```python
from build123d import *

# Parameters (mm, degrees)
SKETCH1_R           = 2.75
BOSS_EXTRUDE1_DEPTH = 6.35


with BuildPart() as part:
    # Sketch1 → Boss-Extrude1 (new body)
    with BuildSketch(Plane.XY):
        Polygon((182, -212), (212, -212), (212, -182), (232.5, -182), (232.5, 0), (232.5, 182), (212, 182), (212, 212), (182, 212), (182, 232.5), (8, 232.5), (8, 191.5), (-48, 191.5), (-48, 232.5), (-182, 232.5), (-182, 212), (-212, 212), (-212, 182), (-232.5, 182), (-232.5, 0), (-232.5, -182), (-212, -182), (-212, -212), (-182, -212), (-182, -232.5), (-8, -232.5), (-8, -191.5), (48, -191.5), (48, -232.5), (182, -232.5), align=None)
        with Locations((-222.5, -162)):
            Circle(SKETCH1_R, mode=Mode.SUBTRACT)
        with Locations(Location((222.5, -162, 0), (0, 0, 180))):
            Circle(SKETCH1_R, mode=Mode.SUBTRACT)
        with Locations((222.5, 162)):
            Circle(SKETCH1_R, mode=Mode.SUBTRACT)
        with Locations(Location((-222.5, 162, 0), (0, 0, 180))):
            Circle(SKETCH1_R, mode=Mode.SUBTRACT)
    extrude(amount=BOSS_EXTRUDE1_DEPTH)


solid = part.part
```
Could you check a few things on this model? Use its own coordinates, in mm. Coordinates: 2 decimals unless noted, no trailing zeros. Loops run counter-clockwise (first coordinate to the right, second up) from the corner with the lowest first, then second, coordinate; pieces in that order, holes last. Notation, with made-up numbers: M 35,64.25 L 93,64.25 A8 cw 93,74.25 Z; hole C -19.75,12.5 d3. An arc over 180 degrees is marked long. Put each result on its own line as item: value. Start each with the question number.
(1) Will these pins go through, and if not, where does the flat tip stop? P1, Ø1.9, axis at x = -6.5, z = 4, coming from the +Y side; P2, Ø3, axis at x = 220, z = 2, coming from the +Y side; P3, Ø2, axis at x = 81.5, y = 181.5, coming from the -Z side; P4, Ø3, axis at y = -206.5, z = 3, coming from the +X side.
(2) Suppose I cut it at B-B on x = 192. Please give me the cut outline in (y, z), then the cut area to 3 significant figures.
(3) I need wall thicknesses on line 1 (Y direction, x = 222.5, z = 3.5); line 2 (X direction, y = 162, z = 4); line 3 (X direction, y = -199, z = 4.5). Which ranges of each line are inside material? Lowest first, please. Write a range as from..to.
(4) Suppose I cut it at C-C on x = 2. Please give me the cut outline in (y, z).
(5) Suppose I cut it at A-A on z = 1.5. Count the separate pieces of the cut face and the enclosed holes in it, then the cut area to 3 significant figures.
Solutions:
1. P1: stops at y = 191.5
1. P2: stops at y = 182
1. P3: stops at z = 0
1. P4: stops at x = 212
2. outline: M -212,0 L 212,0 L 212,6.35 L -212,6.35 Z
2. area: 2,690 mm2
3. line 1: y = -182..-164.75, -159.25..159.25, 164.75..182
3. line 2: x = -232.5..-225.25, -219.75..219.75, 225.25..232.5
3. line 3: x = -212..-8, 48..212
4. outline: M -191.5,0 L 191.5,0 L 191.5,6.35 L -191.5,6.35 Z
5. separate pieces: 1
5. enclosed holes: 4
5. area: 205,000 mm2
